Build history of the part. All positions in model axes, mm. A direction names the side the tool comes from. Give positions to 0.01 mm unless a question says otherwise; leave off trailing zeros. Write each loop counter-clockwise with the first axis right and the second up, starting at its lowest first coordinate (ties: lowest second). Pieces come first, ordered by that corner, then holes. Notation, with made-up numbers: M 24.5,77.5 L 45.5,77.5 A11 ccw 45.5,89.5 Z; hole C -20,29.5 d8. An arc over 180 degrees is marked long. One line per item, written item: value. Start each with the question number.
from build123d import *

# Parameters (mm, degrees)
SKETCH1_W           = 50.8
SKETCH1_H           = 203.2
BOSS_EXTRUDE1_DEPTH = 25.4
SHELL1_T            = -3.175
FILLET1_R           = 6.35


with BuildPart() as part:
    # Sketch1 → Boss-Extrude1 (new body)
    with BuildSketch(Plane(origin=(0, 0, 0), x_dir=(1, 0, 0), z_dir=(0, 1, 0))):
        with Locations((25.4, 101.6)):
            Rectangle(SKETCH1_W, SKETCH1_H)
    extrude(amount=BOSS_EXTRUDE1_DEPTH)

    # Shell1
    shell1_openings = [part.faces().sort_by_distance(p)[0] for p in [
        (25.4, 25.4, -101.6),
    ]]
    offset(amount=SHELL1_T, openings=shell1_openings, kind=Kind.INTERSECTION)

    # Fillet1
    fillet1_edges = [part.edges().sort_by_distance(p)[0] for p in [
        (3.175, 14.2875, -200.025),
        (3.175, 14.2875, -3.175),
        (47.625, 14.2875, -3.175),
        (47.625, 14.2875, -200.025),
    ]]
    fillet(fillet1_edges, radius=FILLET1_R)


solid = part.part
1) Band-saw the part on A-A (x = 13.5). List the corners of the cut face in (y, z) (3 decimals), then the cut area to 3 significant figures.
2) Probe line 1 along X through (y, z) = (15.75, -10) (3 decimals); line 2 along Z through (x, y) = (12, 10.25) (3 decimals); line 3 along Y through (x, z) = (17, -159) (3 decimals). List the from-to ranges inside material, lowest first. Write a range as from..to.
3) Drop a flat-ended pin along its axis: P1, Ø13.5, axis at x = 17.5, z = -137, coming from the +Y side (3 decimals). Give the stop position or say it passes through.
4) Band-saw the part on B-B (z = -34.5). List the corners of the cut face in (x, y) (3 decimals), then the cut area to 3 significant figures.
5) Tool access for faces 1 (the face through (25, 0, -103)), 2 (the face through (25, 3.175, -103)): list every direction of +Z, -Z, +X, -X, +Y, -Y with a clear straight run to the whole face (end or side of a thin tool).
6) Band-saw the part on C-C (y = 20.75). List the corners of the cut face in (x, z) (3 decimals).
7) Mould opens along Z. For faces 3 (the face through (0, 13, -100)), 4 (the face through (25, 13, 0)), 5 (the face through (3.175, 14, -100)), 6 (the face through (4.99, 14.13, -5.08)) say: released by +Z, released by -Z, zero draft, split by the parting line, or undercut.
Model answer:
1. outline: M 0,-203.2 L 25.4,-203.2 L 25.4,-200.025 L 3.175,-200.025 L 3.175,-3.175 L 25.4,-3.175 L 25.4,0 L 0,0 Z
1. area: 786 mm²
2. line 1: x = 0..3.175, 47.625..50.8
2. line 2: z = -203.2..-200.025, -3.175..0
2. line 3: y = 0..3.175
3. P1: stops at y = 3.175
4. outline: M 0,0 L 50.8,0 L 50.8,25.4 L 47.625,25.4 L 47.625,3.175 L 3.175,3.175 L 3.175,25.4 L 0,25.4 Z
4. area: 302 mm²
5. face 1: +Z, -Z, +X, -X, -Y
5. face 2: +Y
6. outline: M 0,-203.2 L 50.8,-203.2 L 50.8,0 L 0,0 Z; hole M 3.175,-193.675 A6.35 ccw 9.525,-200.025 L 41.275,-200.025 A6.35 ccw 47.625,-193.675 L 47.625,-9.525 A6.35 ccw 41.275,-3.175 L 9.525,-3.175 A6.35 ccw 3.175,-9.525 Z
7. face 3: zero draft
7. face 4: released by +Z
7. face 5: undercut
7. face 6: undercut
